Part model, mm, in its own coordinate system. A direction names the side the tool comes from. Coordinates: 2 decimals unless noted, no trailing zeros. Order: outer loops, then holes, each group sorted by start corner. A loop starts at its lowest first (then second) coordinate and runs counter-clockwise, first axis right, second up.
1) Tool access for faces 1 (the flat face through (80, 16, 80)), 2 (the cylindrical face through (121.61, 7.89, 113.86)): list every direction of +Z, -Z, +X, -X, +Y, -Y with a clear straight run to the whole face (end or side of a thin tool).
2) Mould opens along X. For faces 3 (the flat face through (80, 0, -3)), 4 (the cylindrical face through (177.4, 8.1, -55.9)), 5 (the cylindrical face through (-176.494, 7.888, 0.286)), 6 (the cylindrical face through (-14.524, 34.51, -65.407)) say: +X half, -X half, draft (parallel to the pull), parting line (faces both ways), or undercut.
3) Cut at D-D (y = 34). List the corners of the cut face in (x, z).
4) Cut at B-B (x = -170). List the corners of the cut face in (y, z).
5) Cut at A-A (x = 0). List the corners of the cut face in (y, z).
6) Wall check: L1, parallel to X at y = 44, z = 0; L2, parallel to Y at x = 93, z = 61; L3, parallel to Z at x = 61, y = 66.5. Give the ranges that are in metal, low to high.
7) Cut at C-C (z = 62). List the corners of the cut face in (x, y).
8) Pin check, flat tips, straight feed: pin 1 Ø1.5 at (y, z) = (33, -56) entering from +X; pin 2 Ø8 at (x, y) = (27, 47.5) entering from -Z; pin 3 Ø21 at (x, z) = (-120.21, -120.21) entering from +Y; pin 4 Ø10.5 at (x, z) = (-120.21, 120.21) entering from -Y. Stop position of each tip, or through.
Autodesk Inventor part; units mm, degrees
ref_plane "YZ Plane" through (0, 0, 0) normal (1, 0, 0) x (0, 1, 0)
ref_plane "XZ Plane" through (0, 0, 0) normal (0, 1, 0) x (-1, 0, 0)
ref_plane "XY Plane" through (0, 0, 0) normal (0, 0, 1) x (1, 0, 0)
sketch "Sketch2" plane through (0, 0, 0) normal (0, 0, 1) x (1, 0, 0)
  line L0 (67, 70) -> (67, 0)
  line L1 (67, 0) -> (186, 0)
  line L2 (186, 0) -> (186, 16)
  line L3 (186, 16) -> (96, 16)
  line L4 (96, 16) -> (96, 70)
  line L5 (96, 70) -> (67, 70)
  line L6 (0, 0) -> (0, 134.3394)
  dimension "d1" = 70
  dimension "d2" = 119
  dimension "d3" = 29
  dimension "d4" = 134
  dimension "d5" = 16
revolve "Revolution1" add sketch "Sketch2" angle 360 about axis through (0, 0, 0) along (0, 1, 0)
sketch "Sketch3" plane through (0, 16, 0) normal (0, 1, 0) x (1, 0, 0)
  circle A0 centre (0, 0) radius 170 construction
  point P0 (0, 170)
  dimension "d7" = 340
hole "Hole1" at (0, 16, -170) direction (0, -1, 0) diameter 13 end through all
pattern_circular "Circular Pattern1" count 8 over 360 about axis through (0, -10, 0) along (0, 1, 0) of "Hole1"
equation "\"BendRadius\" = Thickness"
equation "\"BendReliefWidth\" = Thickness"
equation "\"BendReliefDepth\" = 0.5 * Thickness"
equation "\"CornerReliefSize\" = 4 * Thickness"
equation "\"MinimumRemnant\" = 2 * Thickness"
equation "\"TransitionRadius\" = BendRadius"
equation "\"JacobiRadiusSize\" = BendRadius"
equation "\"GapSize\" = Thickness"
properties part number "DMF Hat 2.0"
Geometry check:
1. face 1: +Y
1. face 2: +Y, -Y
2. face 3: draft
2. face 4: parting line
2. face 5: undercut
2. face 6: undercut
3. outline: circle Ø192 at (0, 0); hole circle Ø134 at (0, 0)
4. outline: (0, -75.47) - (16, -75.47) - (16, -6.5) - (0, -6.5) - close; (0, 6.5) - (16, 6.5) - (16, 75.47) - (0, 75.47) - close
5. outline: (0, -186) - (16, -186) - (16, -176.5) - (0, -176.5) - close; (0, -163.5) - (16, -163.5) - (16, -96) - (70, -96) - (70, -67) - (0, -67) - close; (0, 67) - (70, 67) - (70, 96) - (16, 96) - (16, 163.5) - (0, 163.5) - close; (0, 176.5) - (16, 176.5) - (16, 186) - (0, 186) - close
6. L1: x = -96 to -67, 67 to 96
6. L2: y = 0 to 16
6. L3: z = -74.13 to -27.71, 27.71 to 74.13
7. outline: (-175.36, 0) - (-25.4, 0) - (-25.4, 70) - (-73.29, 70) - (-73.29, 16) - (-175.36, 16) - close; (25.4, 0) - (175.36, 0) - (175.36, 16) - (73.29, 16) - (73.29, 70) - (25.4, 70) - close
8. pin 1: stops at x = 78.51
8. pin 2: stops at z = -93.2
8. pin 3: stops at y = 16
8. pin 4: passes through
